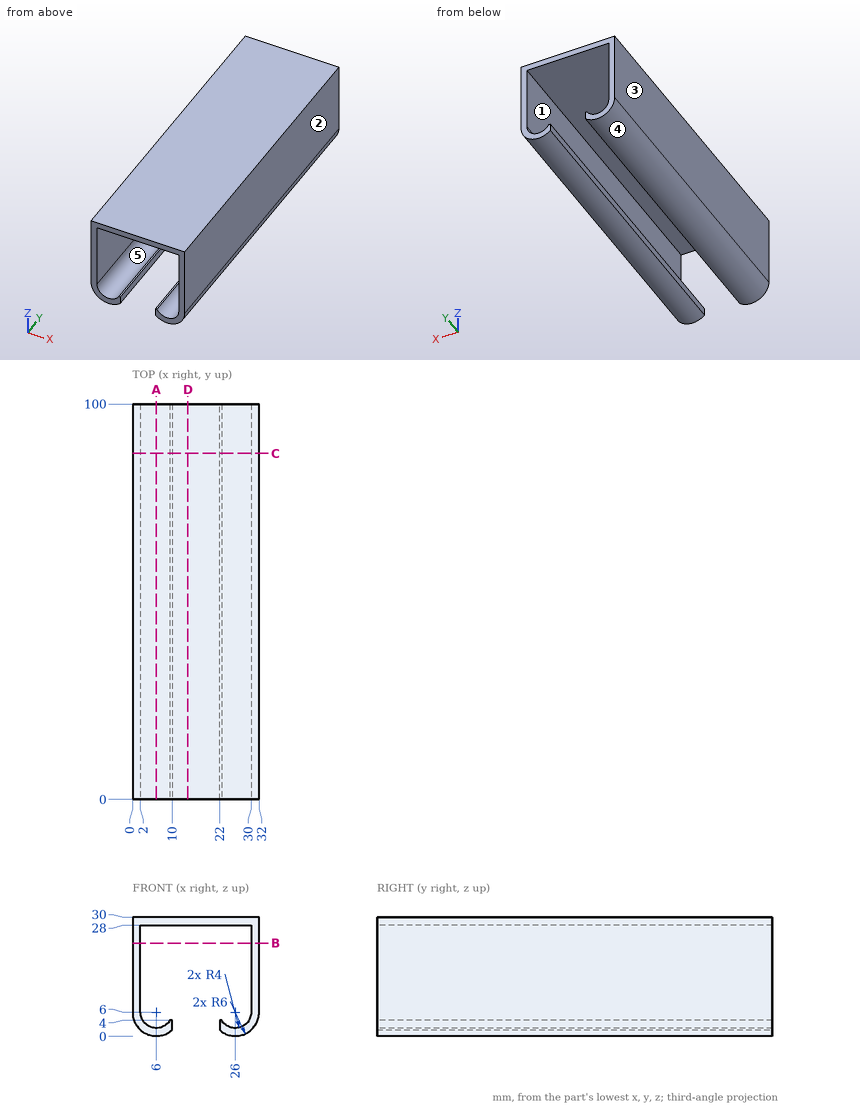
Could you check a few things on this drawing? It's one solid part, dimensions in mm from its lowest x, y, z. A direction names the side the tool comes from. Give positions to 0.01 mm unless a question says otherwise; leave off trailing zeros. Order: outer loops, then holes, each group sorted by start corner. A loop starts at its lowest first (then second) coordinate and runs counter-clockwise, first axis right, second up.
1. Suppose I cut it at A-A (x = 6). Write out the boundary of the cut face in (y, z).
Answers below:
outline: (0, 0) - (100, 0) - (100, 2) - (0, 2) - close; (0, 28) - (100, 28) - (100, 30) - (0, 30) - close
2. Which directions (+Z, -Z, +X, -X, +Y, -Y) give clear straight access to the entire face, cutting with the end or side of a thin tool? Please do the marked faces 4 and 5.
Answers below:
face 4: -Z, +Y, -Y
face 5: +Y, -Y
3. For pin 1 (5 mm diameter, centred on x = 9.5, y = 68.5, fed in from -Z); pin 2 (4 mm diameter, centred on x = 24.5, z = 25, fed in from -Y); pin 3 (1.5 mm diameter, centred on y = 47.5, z = 15, fed in from -X); pin 4 (0.7 mm diameter, centred on y = 43, z = 3, fed in from -X), each with a flat end and sliding along its axis, tell me the tip position at first contact or that it passes through.
Answers below:
pin 1: stops at z = 0.08
pin 2: passes through
pin 3: stops at x = 0
pin 4: stops at x = 0.62
4. Suppose I cut it at D-D (x = 14). Write out the boundary of the cut face in (y, z), plus the area to 3 significant figures.
Answers below:
outline: (0, 28) - (100, 28) - (100, 30) - (0, 30) - close
area: 200 mm2
5. Suppose I cut it at C-C (y = 87.5). Write out the boundary of the cut face in (x, z).
Answers below:
outline: (0, 6) arc R6 ccw to (10, 1.53) - (10, 4) - (9.46, 4) arc R4 cw to (2, 6) - (2, 28) - (30, 28) - (30, 6) arc R4 cw to (22.54, 4) - (22, 4) - (22, 1.53) arc R6 ccw to (32, 6) - (32, 30) - (0, 30) - close
6. I need wall thicknesses on L1, parallel to X at y = 18, z = 24; L2, parallel to Z at x = 12.5, y = 64; L3, parallel to Z at x = 9, y = 54.5. Which ranges of each line are inside material? Lowest first, please.
Answers below:
L1: x = 0 to 2, 30 to 32
L2: z = 28 to 30
L3: z = 0.8 to 3.35, 28 to 30
7. Thinking about a two-plate mould opening in X: for the marked faces 1, 2 and 3, which applies, +X half, -X half, draft (parallel to the pull), parting line (faces both ways), or undercut?
Answers below:
face 1: undercut
face 2: +X half
face 3: -X half
8. Suppose I cut it at B-B (z = 23.5). Write out the boundary of the cut face in (x, y).
Answers below:
outline: (0, 0) - (2, 0) - (2, 100) - (0, 100) - close; (30, 0) - (32, 0) - (32, 100) - (30, 100) - close
